The model under review builds one solid part; all positions refer to its coordinate system, in mm. A direction names the side the tool comes from. Give positions to 0.01 mm unless a question says otherwise; leave off trailing zeros. Use CSV: the item, a comma, the result in double quotes.
```python
from build123d import *

# Parameters (mm, degrees)
EXTRUDE_1_DEPTH = 760


with BuildPart() as part:
    # 草图1 → 凸台-拉伸1 (new body)
    with BuildSketch(Plane.XY):
        with BuildLine():
            Line((-6.089339828, -7.15), (6.089339828, -7.15))
            Line((6.089339828, -7.15), (7.15, -8.210660172))
            Line((7.15, -8.210660172), (7.15, -18.5))
            Line((7.15, -18.5), (4.2, -18.5))
            Line((4.2, -18.5), (4.2, -20))
            Line((4.2, -20), (18.5, -20))
            ThreePointArc((18.5, -20), (19.560660172, -19.560660172), (20, -18.5))
            Line((20, -18.5), (20, -4.2))
            Line((20, -4.2), (18.5, -4.2))
            Line((18.5, -4.2), (18.5, -7.15))
            Line((18.5, -7.15), (8.210660172, -7.15))
            Line((8.210660172, -7.15), (7.15, -6.089339828))
            Line((7.15, -6.089339828), (7.15, 6.089339828))
            Line((7.15, 6.089339828), (8.210660172, 7.15))
            Line((8.210660172, 7.15), (18.5, 7.15))
            Line((18.5, 7.15), (18.5, 4.2))
            Line((18.5, 4.2), (20, 4.2))
            Line((20, 4.2), (20, 18.5))
            ThreePointArc((20, 18.5), (19.560660172, 19.560660172), (18.5, 20))
            Line((18.5, 20), (4.2, 20))
            Line((4.2, 20), (4.2, 18.5))
            Line((4.2, 18.5), (7.15, 18.5))
            Line((7.15, 18.5), (7.15, 8.210660172))
            Line((7.15, 8.210660172), (6.089339828, 7.15))
            Line((6.089339828, 7.15), (-6.089339828, 7.15))
            Line((-6.089339828, 7.15), (-7.15, 8.210660172))
            Line((-7.15, 8.210660172), (-7.15, 18.5))
            Line((-7.15, 18.5), (-4.2, 18.5))
            Line((-4.2, 18.5), (-4.2, 20))
            Line((-4.2, 20), (-18.5, 20))
            ThreePointArc((-18.5, 20), (-19.560660172, 19.560660172), (-20, 18.5))
            Line((-20, 18.5), (-20, 4.2))
            Line((-20, 4.2), (-18.5, 4.2))
            Line((-18.5, 4.2), (-18.5, 7.15))
            Line((-18.5, 7.15), (-8.210660172, 7.15))
            Line((-8.210660172, 7.15), (-7.15, 6.089339828))
            Line((-7.15, 6.089339828), (-7.15, -6.089339828))
            Line((-7.15, -6.089339828), (-8.210660172, -7.15))
            Line((-8.210660172, -7.15), (-18.5, -7.15))
            Line((-18.5, -7.15), (-18.5, -4.2))
            Line((-18.5, -4.2), (-20, -4.2))
            Line((-20, -4.2), (-20, -18.5))
            ThreePointArc((-20, -18.5), (-19.560660172, -19.560660172), (-18.5, -20))
            Line((-18.5, -20), (-4.2, -20))
            Line((-4.2, -20), (-4.2, -18.5))
            Line((-4.2, -18.5), (-7.15, -18.5))
            Line((-7.15, -18.5), (-7.15, -8.210660172))
            Line((-7.15, -8.210660172), (-6.089339828, -7.15))
        make_face()
        with BuildLine():
            Line((17.4, 8.25), (9.75, 8.25))
            ThreePointArc((9.75, 8.25), (8.689339828, 8.689339828), (8.25, 9.75))
            Line((8.25, 9.75), (8.25, 17.4))
            ThreePointArc((8.25, 17.4), (8.689339828, 18.460660172), (9.75, 18.9))
            Line((9.75, 18.9), (17.4, 18.9))
            ThreePointArc((17.4, 18.9), (18.460660172, 18.460660172), (18.9, 17.4))
            Line((18.9, 17.4), (18.9, 9.75))
            ThreePointArc((18.9, 9.75), (18.460660172, 8.689339828), (17.4, 8.25))
        make_face(mode=Mode.SUBTRACT)
        with BuildLine():
            Line((-8.25, 17.4), (-8.25, 9.75))
            ThreePointArc((-8.25, 9.75), (-8.689339828, 8.689339828), (-9.75, 8.25))
            Line((-9.75, 8.25), (-17.4, 8.25))
            ThreePointArc((-17.4, 8.25), (-18.460660172, 8.689339828), (-18.9, 9.75))
            Line((-18.9, 9.75), (-18.9, 17.4))
            ThreePointArc((-18.9, 17.4), (-18.460660172, 18.460660172), (-17.4, 18.9))
            Line((-17.4, 18.9), (-9.75, 18.9))
            ThreePointArc((-9.75, 18.9), (-8.689339828, 18.460660172), (-8.25, 17.4))
        make_face(mode=Mode.SUBTRACT)
        with BuildLine():
            Line((-17.4, -8.25), (-9.75, -8.25))
            ThreePointArc((-9.75, -8.25), (-8.689339828, -8.689339828), (-8.25, -9.75))
            Line((-8.25, -9.75), (-8.25, -17.4))
            ThreePointArc((-8.25, -17.4), (-8.689339828, -18.460660172), (-9.75, -18.9))
            Line((-9.75, -18.9), (-17.4, -18.9))
            ThreePointArc((-17.4, -18.9), (-18.460660172, -18.460660172), (-18.9, -17.4))
            Line((-18.9, -17.4), (-18.9, -9.75))
            ThreePointArc((-18.9, -9.75), (-18.460660172, -8.689339828), (-17.4, -8.25))
        make_face(mode=Mode.SUBTRACT)
        with BuildLine():
            Line((8.25, -17.4), (8.25, -9.75))
            ThreePointArc((8.25, -9.75), (8.689339828, -8.689339828), (9.75, -8.25))
            Line((9.75, -8.25), (17.4, -8.25))
            ThreePointArc((17.4, -8.25), (18.460660172, -8.689339828), (18.9, -9.75))
            Line((18.9, -9.75), (18.9, -17.4))
            ThreePointArc((18.9, -17.4), (18.460660172, -18.460660172), (17.4, -18.9))
            Line((17.4, -18.9), (9.75, -18.9))
            ThreePointArc((9.75, -18.9), (8.689339828, -18.460660172), (8.25, -17.4))
        make_face(mode=Mode.SUBTRACT)
        with BuildLine():
            Line((-4.243347723, 2.829134161), (-5.656854249, 4.242640687))
            ThreePointArc((-5.656854249, 4.242640687), (-5.656854249, 5.656854249), (-4.242640687, 5.656854249))
            Line((-4.242640687, 5.656854249), (-2.829134161, 4.243347723))
            ThreePointArc((-2.829134161, 4.243347723), (0, 5.1), (2.829134161, 4.243347723))
            Line((2.829134161, 4.243347723), (4.242640687, 5.656854249))
            ThreePointArc((4.242640687, 5.656854249), (5.656854249, 5.656854249), (5.656854249, 4.242640687))
            Line((5.656854249, 4.242640687), (4.243347723, 2.829134161))
            ThreePointArc((4.243347723, 2.829134161), (5.1, 0), (4.243347723, -2.829134161))
            Line((4.243347723, -2.829134161), (5.656854249, -4.242640687))
            ThreePointArc((5.656854249, -4.242640687), (5.656854249, -5.656854249), (4.242640687, -5.656854249))
            Line((4.242640687, -5.656854249), (2.829134161, -4.243347723))
            ThreePointArc((2.829134161, -4.243347723), (0, -5.1), (-2.829134161, -4.243347723))
            Line((-2.829134161, -4.243347723), (-4.242640687, -5.656854249))
            ThreePointArc((-4.242640687, -5.656854249), (-5.656854249, -5.656854249), (-5.656854249, -4.242640687))
            Line((-5.656854249, -4.242640687), (-4.243347723, -2.829134161))
            ThreePointArc((-4.243347723, -2.829134161), (-5.1, 0), (-4.243347723, 2.829134161))
        make_face(mode=Mode.SUBTRACT)
    extrude(amount=EXTRUDE_1_DEPTH)


solid = part.part
```
Q1. To check wall thickness, follow probe 1 along X at (y, z) = (-15.5, 185); probe 2 along X at (y, z) = (-6, 492); probe 3 along X at (y, z) = (18, 662). State the ranges of each line that lie inside material, in increasing order.
Derived:
probe 1,"x = -20 to -18.9, -8.25 to -7.15, 7.15 to 8.25, 18.9 to 20"
probe 2,"x = -20 to -18.5, -7.15 to 7.15, 18.5 to 20"
probe 3,"x = -20 to -18.77, -8.38 to -7.15, 7.15 to 8.38, 18.77 to 20"
Q2. Machinability: for faces 5 (the flat face through (0, -7.15, 375)), 6 (the flat face through (-20, 11, 375)), which of the approach directions +Z, -Z, +X, -X, +Y, -Y give a long, thin tool a straight path to every point of the face, cutting with its end or side? Answer none if there is none.
Derived:
face 5,"+Z, -Z"
face 6,"+Z, -Z, -X, +Y, -Y"
Q3. Consider section A-A (z = 534.5). State how many separate pieces and enclosed holes the cut face has, then the cut area to 3 significant figures.
Derived:
separate pieces,"1"
enclosed holes,"5"
area,"354 mm2"
Q4. The part is to be moulded in two halves that separate along X. For faces 1 (the flat face through (-20, -11, 375)), 2 (the flat face through (-7.15, 0, 375)), 3 (the flat face through (20, 11, 375)), 4 (the flat face through (-5, -3, 760)), say which applies: pulls with the +X half, pulls with the -X half, needs draft (parallel to the pull), parting line crosses it, or undercut.
Derived:
face 1,"pulls with the -X half"
face 2,"undercut"
face 3,"pulls with the +X half"
face 4,"needs draft"
Q5. Insertion check: pin 1 (1.6 mm diameter, centred on x = 19, z = 554, fed in from +Y); pin 2 (3 mm diameter, centred on x = 2.5, z = 381, fed in from +Y). Each pin has a flat end and moves straight along its axis. Give the tip position at first contact, or say it passes through.
Derived:
pin 1,"stops at y = 20"
pin 2,"stops at y = 7.15"
